from build123d import *

# Parameters (mm, degrees)
SKETCH1_R           = 25
BOSS_EXTRUDE1_DEPTH = 9
SHELL1_T            = -1
FILLET1_R           = 0.5
FILLET2_R           = 1.5


with BuildPart() as part:
    # Sketch1 → Boss-Extrude1 (new body)
    with BuildSketch(Plane.XY):
        Circle(SKETCH1_R)
    extrude(amount=BOSS_EXTRUDE1_DEPTH)

    # Shell1
    shell1_openings = [part.faces().sort_by_distance(p)[0] for p in [
        (0, 0, 9),
    ]]
    offset(amount=SHELL1_T, openings=shell1_openings, kind=Kind.INTERSECTION)

    # Fillet1
    fillet1_edges = [part.edges().sort_by_distance(p)[0] for p in [
        (-24, 0, 1),
    ]]
    fillet(fillet1_edges, radius=FILLET1_R)

    # Fillet2
    fillet2_edges = [part.edges().sort_by_distance(p)[0] for p in [
        (-25, 0, 0),
    ]]
    fillet(fillet2_edges, radius=FILLET2_R)


solid = part.part
Could you check a few things on this model? Use its own coordinates, in mm. A direction names the side the tool comes from. Give positions to 0.01 mm unless a question says otherwise; leave off trailing zeros. Order: outer loops, then holes, each group sorted by start corner. A loop starts at its lowest first (then second) coordinate and runs counter-clockwise, first axis right, second up. Notation, with made-up numbers: (74, 43) - (118, 43) arc R23 ccw to (118, 63) - close; hole circle Ø3 at (-2, 4.25). An arc over 180 degrees is marked (long way). One line per item, written item: value. Start each with the question number.
1. For faces 1 (the face through (0, 0, 1)), 2 (the face through (-9.4, 22.3, 9)), which set-ups out of +Z, -Z, +X, -X, +Y, -Y let a thin tool reach every point of the face, with its end or its side?
2. For P1, Ø5, axis at x = -20, z = 6.5, coming from the -Y side; P2, Ø14, axis at x = -6, y = -10.5, coming from the +Z side; P3, Ø5, axis at y = 14.5, z = 3.5, coming from the -X side, each with a flat end and sliding along its axis, tell me the tip position at first contact or that it passes through.
3. Imagine slicing it at A-A on y = 0. List the corners of the cut face in (x, z) for me.
4. Imagine slicing it at B-B on z = 4.25. List the corners of the cut face in (x, y) for me, plus the area to 3 significant figures.
5. If I drill on probe 1 along Y at (x, z) = (0, 5.5); probe 2 along Z at (x, y) = (-6.5, 6); probe 3 along X at (y, z) = (2, 2), over which ranges is the centre line in solid material (lowest first)?
Values:
1. face 1: +Z
1. face 2: +Z, +X, -X, +Y, -Y
2. P1: y = -17.85
2. P2: z = 1
2. P3: x = -21.93
3. outline: (-25, 1.5) arc R1.5 ccw to (-23.5, 0) - (23.5, 0) arc R1.5 ccw to (25, 1.5) - (25, 9) - (24, 9) - (24, 1.5) arc R0.5 cw to (23.5, 1) - (-23.5, 1) arc R0.5 cw to (-24, 1.5) - (-24, 9) - (-25, 9) - close
4. outline: circle Ø50 at (0, 0); hole circle Ø48 at (0, 0)
4. area: 154 mm²
5. probe 1: -25 to -24, 24 to 25
5. probe 2: 0 to 1
5. probe 3: -24.92 to -23.92, 23.92 to 24.92
